Verification items for the finished model (mm, model axes). A direction names the side the tool comes from. Coordinates: 2 decimals unless noted, no trailing zeros. Write each loop counter-clockwise with the first axis right and the second up, starting at its lowest first coordinate (ties: lowest second). Pieces come first, ordered by that corner, then holes. Notation, with made-up numbers: (-30, 30) -> (-12, 30) arc R21 cw to (-12, 68) -> close; hole circle Ø5 at (48.5, -7.5). An arc over 180 degrees is marked (long way). Write item = value, one per line. Start each with the question number.
(1) Set-up check for faces 1 (the face through (-52, 97, -132)), 2 (the face through (-12, 96, -136)), 3 (the face through (-55, 98, -133)), 4 (the face through (-8, 98, -133)): record each of +Z, -Z, +X, -X, +Y, -Y from which the full face is reachable in a straight line by a thin tool's end or side.
(2) Section check B-B (z = -62). Record the cut outline in (x, y).
(3) Material ranges on probe 1 along Y at (x, z) = (-49, -119), recorded low to high. Write a range as [from, to].
(4) Mould release check, pull along Y, two halves, no side actions. Record for faces 5 (the face through (-52, 99, -133)), 6 (the face through (-11, 97, -132)), 7 (the face through (-63, 46, -75)): released by +Y, released by -Y, zero draft, split by the parting line, or undercut.
(5) Gauge pin test, flat ends, axial feed: pin 1 Ø5.5 at (x, y) = (-51.5, 97.5) entering from -Z; pin 2 Ø1.5 at (y, z) = (95.5, -131.5) entering from -X; pin 3 Ø5.5 at (y, z) = (97, -133) entering from -X; pin 4 Ø2 at (x, y) = (-51.5, 98) entering from +Z. Record the tip position at first contact, or that the pin passes through.
(6) Section check A-A (x = -38). Record the cut outline in (y, z).
Autodesk Inventor part; units mm, degrees
ref_plane "YZ Plane" through (0, 0, 0) normal (1, 0, 0) x (0, 1, 0)
ref_plane "XZ Plane" through (0, 0, 0) normal (0, 1, 0) x (-1, 0, 0)
ref_plane "XY Plane" through (0, 0, 0) normal (0, 0, 1) x (1, 0, 0)
sketch "Sketch1" plane through (0, 0, 0) normal (0, 1, 0) x (-1, 0, 0)
  line L0 (0, 0) -> (0, -148)
  line L1 (0, -148) -> (63, -148)
  line L2 (63, -148) -> (63, 0)
  line L3 (63, 0) -> (0, 0)
  dimension "d0" = 148
  dimension "d1" = 63
extrude "Extrusion1" add sketch "Sketch1" along normal blind 94
sketch "Sketch2" plane through (0, 94, 0) normal (0, 1, 0) x (1, 0, 0)
  line L0 (0, 148) -> (-63, 148)
  line L1 (-63, 148) -> (-63, 136)
  line L2 (-63, 148) -> (-63, 0)
  line L3 (-63, 136) -> (-55, 136)
  line L4 (-55, 136) -> (-48, 136)
  line L5 (-48, 136) -> (-48, 134)
  line L6 (-48, 134) -> (-55, 134)
  line L7 (-55, 134) -> (-55, 136)
  line L8 (0, 0) -> (0, 148)
  line L9 (0, 148) -> (0, 136)
  line L10 (0, 136) -> (-8, 136)
  line L11 (-8, 136) -> (-8, 134)
  line L12 (-8, 134) -> (-15, 134)
  line L13 (-15, 134) -> (-15, 136)
  line L14 (-15, 136) -> (-8, 136)
  dimension "d4" = 12
  dimension "d5" = 8
  dimension "d6" = 7
  dimension "d7" = 2
  dimension "d8" = 12
  dimension "d9" = 8
  dimension "d10" = 2
  dimension "d11" = 7
extrude "Extrusion2" add sketch "Sketch2" along normal blind 5
sketch "Sketch3" plane through (-55, 94, -134) normal (0, 0, 1) x (1, 0, 0)
  line L0 (0, 5) -> (7, 5)
  line L1 (0, 5) -> (0, 3)
  line L2 (0, 0) -> (0, 5)
  line L3 (0, 3) -> (7, 3)
  line L4 (7, 0) -> (7, 5)
  line L5 (7, 5) -> (0, 5)
  line L6 (7, 5) -> (7, 3)
  line L7 (40, 5) -> (47, 5)
  line L8 (40, 5) -> (47, 5)
  line L9 (47, 5) -> (47, 3)
  line L10 (47, 0) -> (47, 5)
  line L11 (47, 3) -> (40, 3)
  line L12 (40, 0) -> (40, 5)
  line L13 (40, 5) -> (40, 3)
  point P0 (55, -94)
  dimension "d14" = 2
  dimension "d15" = 2
extrude "Extrusion3" add sketch "Sketch3" along normal blind 5
fillet "Fillet1" radius 2 12 edges at (0, 94, -74) (-63, 94, -74) (-31.5, 94, -148) (0, 47, -148) (-63, 47, -148) (0, 0, -74) (-31.5, 0, -148) (0, 47, 0) (-31.5, 94, 0) (-63, 47, 0) (-31.5, 0, 0) (-63, 0, -74)
properties part number "battery"
Response:
q1.face_1 = +Z, +X, -X
q1.face_2 = -Z, +X, -X, +Y
q1.face_3 = +Z, -Z, -X, +Y
q1.face_4 = +Z, -Z, +X, +Y
q2.outline = (-63, 2) arc R2 ccw to (-61, 0) -> (-2, 0) arc R2 ccw to (0, 2) -> (0, 92) arc R2 ccw to (-2, 94) -> (-61, 94) arc R2 ccw to (-63, 92) -> close
q3.probe_1 = [0, 94]
q4.face_5 = released by +Y
q4.face_6 = undercut
q4.face_7 = zero draft
q5.pin_1 = -136
q5.pin_2 = through
q5.pin_3 = -55
q5.pin_4 = -129
q6.outline = (0, -146) arc R2 ccw to (2, -148) -> (92, -148) arc R2 ccw to (94, -146) -> (94, -2) arc R2 ccw to (92, 0) -> (2, 0) arc R2 ccw to (0, -2) -> close
